CAD build for the part. Positions are in the model's coordinates, mm. Face numbers are marked on the shaded views. A direction names the side the tool comes from. Coordinates: 2 decimals unless noted, no trailing zeros. Write each loop counter-clockwise with the first axis right and the second up, starting at its lowest first coordinate (ties: lowest second). Pieces come first, ordered by that corner, then holes. Notation, with made-up numbers: (66.25, -33) - (83.25, -33) arc R27 cw to (83.25, -5) - close; hole circle Ø6 at (79.25, 78.25). An arc over 180 degrees is marked (long way). One line per question, with ' | ' between items. Start each with the question number.
1. Which spindle directions (+Z, -Z, +X, -X, +Y, -Y) get a long thin tool onto all of the face, cutting with end or side? Do the marked faces 4, 5 and 6. Say none if no direction does.
2. Two-plate mould, pull along Y, no slides. Class the marked faces 1, 2 and 3: +Y half, -Y half, draft (parallel to the pull), parting line (faces both ways), or undercut.
3. Band-saw the part on D-D, the plane x = 38. Write the cut outline in (y, z).
4. Probe line 1 (X direction, y = 0, z = 80.5). List the from-to ranges inside material, lowest first.
5. Flat gauge pins, fed straight in: P1, Ø8, axis at x = -24.5, y = -44.5, coming from the +Z side; P2, Ø1, axis at y = -46.5, z = 57.5, coming from the +X side; P3, Ø2, axis at x = -41, y = -25, coming from the -Z side. Where does each tip first touch, or does it go through?
6. Band-saw the part on A-A, the plane x = 0. Give the number of separate pieces and of enclosed holes in the cut face, then the cut area to 3 significant figures.
7. Band-saw the part on C-C, the plane z = -23. Write the cut outline in (x, y), then the cut area to 3 significant figures.
from build123d import *

# Parameters (mm, degrees)
SKETCH1_R                = 50.8
BOSS_EXTRUDE1_DEPTH      = 123.698
SKETCH31_R               = 31.75
BOSS_EXTRUDE6_DEPTH      = 87.122
SKETCH7_R                = 31.75
BOSS_EXTRUDE3_DEPTH      = 87.122
BOSS_EXTRUDE3_DEPTH_BACK = 87.122
SKETCH9_R                = 31.75
BOSS_EXTRUDE4_DEPTH      = 87.122
SKETCH11_R               = 19.05
BOSS_EXTRUDE5_DEPTH      = 83.82
SKETCH12_R               = 47.752
CUT_EXTRUDE4_DEPTH       = 124.6980001
SKETCH32_R               = 28.702
CUT_EXTRUDE8_DEPTH       = 88.1220001
SKETCH13_R               = 28.702
CUT_EXTRUDE5_DEPTH       = 88.122
CUT_EXTRUDE5_DEPTH_BACK  = 88.122
SKETCH14_R               = 28.702
CUT_EXTRUDE6_DEPTH       = 88.122
SKETCH15_R               = 17.399
CUT_EXTRUDE7_DEPTH       = 84.82


with BuildPart() as part:
    # Sketch1 → Boss-Extrude1 (new body)
    with BuildSketch(Plane(origin=(0, 0, 0), x_dir=(1, 0, 0), z_dir=(0, 1, 0))):
        Circle(SKETCH1_R)
    extrude(amount=BOSS_EXTRUDE1_DEPTH)

    # Sketch31 → Boss-Extrude6 (add)
    with BuildSketch(Plane(origin=(0, 0, 0), x_dir=(1, 0, 0), z_dir=(0, 1, 0))):
        Circle(SKETCH31_R)
    extrude(amount=-BOSS_EXTRUDE6_DEPTH)

    # Sketch7 → Boss-Extrude3 (add, two sides)
    with BuildSketch(Plane.XY) as boss_extrude3_sk:
        Circle(SKETCH7_R)
    extrude(amount=BOSS_EXTRUDE3_DEPTH)
    extrude(boss_extrude3_sk.sketch, amount=-BOSS_EXTRUDE3_DEPTH_BACK)

    # Sketch9 → Boss-Extrude4 (add)
    with BuildSketch(Plane(origin=(0, 0, 0), x_dir=(0, 0, -1), z_dir=(1, 0, 0))):
        Circle(SKETCH9_R)
    extrude(amount=BOSS_EXTRUDE4_DEPTH)

    # Sketch11 → Boss-Extrude5 (add)
    with BuildSketch(Plane(origin=(0, 0, 0), x_dir=(0, 0, -1), z_dir=(1, 0, 0))):
        Circle(SKETCH11_R)
    extrude(amount=-BOSS_EXTRUDE5_DEPTH)

    # Sketch23 → Revolve-Thin2 (revolve)
    with BuildSketch(Plane(origin=(0, 0, 0), x_dir=(1, 0, 0), z_dir=(0, 1, 0))):
        with BuildLine():
            ThreePointArc((-79.375, 0), (0, 79.375), (79.375, 0))
            Line((79.375, 0), (69.375, 0))
            ThreePointArc((69.375, 0), (0, 69.375), (-69.375, 0))
            Line((-69.375, 0), (-79.375, 0))
        make_face()
    revolve(axis=Axis((79.375, 0, 0), (-1, 0, 0)))

    # Sketch12 → Cut-Extrude4 (cut, through all)
    with BuildSketch(Plane(origin=(0, 0, 0), x_dir=(1, 0, 0), z_dir=(0, 1, 0))):
        Circle(SKETCH12_R)
    extrude(amount=CUT_EXTRUDE4_DEPTH, mode=Mode.SUBTRACT)

    # Sketch32 → Cut-Extrude8 (cut, through all)
    with BuildSketch(Plane(origin=(0, 0, 0), x_dir=(1, 0, 0), z_dir=(0, 1, 0))):
        Circle(SKETCH32_R)
    extrude(amount=-CUT_EXTRUDE8_DEPTH, mode=Mode.SUBTRACT)

    # Sketch13 → Cut-Extrude5 (cut, two sides)
    with BuildSketch(Plane.XY) as cut_extrude5_sk:
        Circle(SKETCH13_R)
    extrude(amount=CUT_EXTRUDE5_DEPTH, mode=Mode.SUBTRACT)
    extrude(cut_extrude5_sk.sketch, amount=-CUT_EXTRUDE5_DEPTH_BACK, mode=Mode.SUBTRACT)

    # Sketch14 → Cut-Extrude6 (cut, through all)
    with BuildSketch(Plane(origin=(0, 0, 0), x_dir=(0, 0, -1), z_dir=(1, 0, 0))):
        Circle(SKETCH14_R)
    extrude(amount=CUT_EXTRUDE6_DEPTH, mode=Mode.SUBTRACT)

    # Sketch15 → Cut-Extrude7 (cut, through all)
    with BuildSketch(Plane(origin=(0, 0, 0), x_dir=(0, 0, -1), z_dir=(1, 0, 0))):
        Circle(SKETCH15_R)
    extrude(amount=-CUT_EXTRUDE7_DEPTH, mode=Mode.SUBTRACT)

    # Sketch26 → Cut-Revolve1 (revolve, cut)
    with BuildSketch(Plane(origin=(0, 0, 0), x_dir=(1, 0, 0), z_dir=(0, 1, 0))):
        with BuildLine():
            Line((0, 76.327), (0, -76.327))
            ThreePointArc((0, -76.327), (76.327, 0), (0, 76.327))
        make_face()
    revolve(axis=Axis((0, 0, -76.327), (0, 0, 1)), mode=Mode.SUBTRACT)


solid = part.part
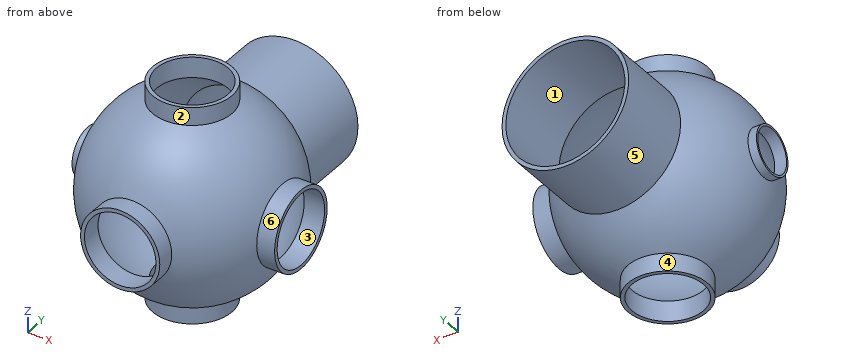
Filled in:
1) face 4: -Z | face 5: +Y | face 6: +X
2) face 1: draft | face 2: parting line | face 3: undercut
3) outline: (59.54, -28.92) arc R66.2 cw (long way) to (59.54, 28.92) - (123.7, 28.92) - (123.7, 33.71) - (60.99, 33.71) arc R69.69 ccw (long way) to (60.99, -33.71) - (123.7, -33.71) - (123.7, -28.92) - close
4) line 1: x = -31.75 to -28.7, 28.7 to 31.75
5) P1: stops at z = 64.11 | P2: stops at x = 30.09 | P3: stops at z = -63.95
6) separate pieces: 4 | enclosed holes: 0 | area: 1,270 mm²
7) outline: (-45.3, 60.99) arc R75.97 ccw to (-21.89, -72.75) - (-21.89, -87.12) - (-17.17, -87.12) - (-17.17, -70.72) arc R72.78 cw to (-41.85, 59.54) - (-41.85, 123.7) - (-45.3, 123.7) - close; (17.17, -87.12) - (21.89, -87.12) - (21.89, -72.75) arc R75.97 ccw to (72.75, -21.89) - (87.12, -21.89) - (87.12, -17.17) - (70.72, -17.17) arc R72.78 cw to (17.17, -70.72) - close; (41.85, 59.54) arc R72.78 cw to (70.72, 17.17) - (87.12, 17.17) - (87.12, 21.89) - (72.75, 21.89) arc R75.97 ccw to (45.3, 60.99) - (45.3, 123.7) - (41.85, 123.7) - close | area: 1,670 mm²
